```python
from build123d import *

# Parameters (mm, degrees)
SKETCH1_W         = 27
SKETCH1_H         = 27
PCB_DEPTH         = 1.2
GLASS_START       = 1.2
SKETCH2_W         = 26
SKETCH2_H         = 15
GLASS_DEPTH       = 1.5
ACTIVE_AREA_START = 2.7
SKETCH3_W         = 22
SKETCH3_H         = 11
ACTIVE_AREA_DEPTH = 0.2
HEADER_START      = 1.2
SKETCH4_W         = 10
SKETCH4_H         = 2.5
HEADER_DEPTH      = 2.5


with BuildPart() as part:
    # Sketch1 → PCB (new body)
    with BuildSketch(Plane(origin=(0, 0, 0), x_dir=(1, 0, 0), z_dir=(0, 1, 0))):
        Rectangle(SKETCH1_W, SKETCH1_H)
    extrude(amount=PCB_DEPTH)

    # Sketch2 → Glass (add)
    with BuildSketch(Plane(origin=(0, 0, 0), x_dir=(1, 0, 0), z_dir=(0, 1, 0)).offset(GLASS_START)):
        Rectangle(SKETCH2_W, SKETCH2_H)
    extrude(amount=GLASS_DEPTH)

    # Sketch3 → Active_Area (add)
    with BuildSketch(Plane(origin=(0, 0, 0), x_dir=(1, 0, 0), z_dir=(0, 1, 0)).offset(ACTIVE_AREA_START)):
        Rectangle(SKETCH3_W, SKETCH3_H)
    extrude(amount=ACTIVE_AREA_DEPTH)

    # Sketch4 → Header (add)
    with BuildSketch(Plane(origin=(0, 0, 0), x_dir=(1, 0, 0), z_dir=(0, 1, 0)).offset(HEADER_START)):
        with Locations((0, -11.5)):
            Rectangle(SKETCH4_W, SKETCH4_H)
    extrude(amount=HEADER_DEPTH)


solid = part.part
```
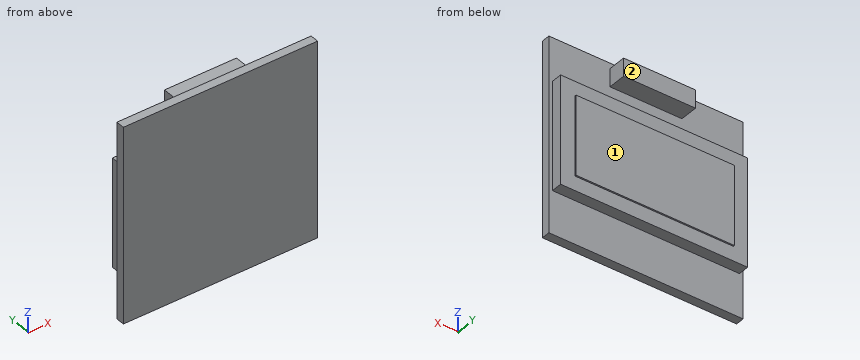
Geometry check sheet. Reference: the model listing, model coordinates, mm. Face numbers are marked on the shaded views. A direction names the side the tool comes from. Coordinates: 2 decimals unless noted, no trailing zeros. Order: outer loops, then holes, each group sorted by start corner. A loop starts at its lowest first (then second) coordinate and runs counter-clockwise, first axis right, second up.
Item 1: Section check D-D (x = -5.5). Enter the section's corners in (y, z).
Item 2: Section check C-C (z = 6.25). Enter the section's corners in (x, y), plus the area to 3 significant figures.
Item 3: Scan lines: line 1 along Z through (x, y) = (0.5, 1.55); line 2 along Y through (x, z) = (-3, 0.5); line 3 along X through (y, z) = (1.25, -2.75). Record each from-to range of solid material in increasing order.
Item 4: Section check A-A (y = 2.35). Enter the section's corners in (x, z), plus the area to 3 significant figures.
Item 5: Depth check by flat-ended pin: pin 1 (2 mm diameter, centred on x = 5.5, z = -5.5, fed in from +Y); pin 2 (2 mm diameter, centred on y = 3, z = 11.5, fed in from +X); pin 3 (0.5 mm diameter, centred on y = 2, z = 3, fed in from -X). Enter the tip coordinate at first touch or a pass-through.
Item 6: Tool access check on the marked faces 1 and 2. Record the directions out of +Z, -Z, +X, -X, +Y, -Y that give a thin tool (end or side, any length) a straight path to the whole face; none if there is none.
Item 7: Section check B-B (x = -2.75). Enter the section's corners in (y, z).
Check sheet entries:
1. outline: (0, -13.5) - (1.2, -13.5) - (1.2, -7.5) - (2.7, -7.5) - (2.7, -5.5) - (2.9, -5.5) - (2.9, 5.5) - (2.7, 5.5) - (2.7, 7.5) - (1.2, 7.5) - (1.2, 13.5) - (0, 13.5) - close
2. outline: (-13.5, 0) - (13.5, 0) - (13.5, 1.2) - (13, 1.2) - (13, 2.7) - (-13, 2.7) - (-13, 1.2) - (-13.5, 1.2) - close
2. area: 71.4 mm2
3. line 1: z = -7.5 to 7.5, 10.25 to 12.75
3. line 2: y = 0 to 2.9
3. line 3: x = -13 to 13
4. outline: (-13, -7.5) - (13, -7.5) - (13, 7.5) - (-13, 7.5) - close; (-5, 10.25) - (5, 10.25) - (5, 12.75) - (-5, 12.75) - close
4. area: 415 mm2
5. pin 1: stops at y = 2.9
5. pin 2: stops at x = 5
5. pin 3: stops at x = -13
6. face 1: -Z, +X, -X, +Y
6. face 2: +Z, -Z, +X, -X, +Y
7. outline: (0, -13.5) - (1.2, -13.5) - (1.2, -7.5) - (2.7, -7.5) - (2.7, -5.5) - (2.9, -5.5) - (2.9, 5.5) - (2.7, 5.5) - (2.7, 7.5) - (1.2, 7.5) - (1.2, 10.25) - (3.7, 10.25) - (3.7, 12.75) - (1.2, 12.75) - (1.2, 13.5) - (0, 13.5) - close
